```python
from build123d import *

# Parameters (mm, degrees)
SKETCH_1_W          = 145
SKETCH_1_H          = 130
SKETCH_1_R          = 2.25
SKETCH_1_W_2        = 31
SKETCH_1_H_2        = 16
EXTRUDE_1_DEPTH     = 2
SKETCH_2_R          = 0.5
SKETCH_2_R_2        = 0.8
CUT_EXTRUDE_1_DEPTH = 2
SKETCH_3_R          = 1
SKETCH_3_R_2        = 4
SKETCH_3_R_3        = 0.9
CUT_EXTRUDE_2_DEPTH = 2
SKETCH_4_R          = 7.5
SKETCH_4_R_2        = 2.5
SKETCH_4_W          = 29
SKETCH_4_H          = 5
EXTRUDE_2_DEPTH     = 8
SKETCH_5_R          = 0.55
SKETCH_5_R_2        = 0.25
CUT_EXTRUDE_3_DEPTH = 10
SKETCH_6_W          = 27
SKETCH_6_H          = 15
SKETCH_6_W_2        = 7.5
SKETCH_6_H_2        = 18
EXTRUDE_3_DEPTH     = 15
SKETCH_7_W          = 27
SKETCH_7_H          = 15
EXTRUDE_4_DEPTH     = 12
SKETCH_9_R          = 0.3
EXTRUDE_5_DEPTH     = 6.5
EXTRUDE_6_DEPTH     = 0.5
SKETCH_11_R         = 2.45
EXTRUDE_7_DEPTH     = 8.5
CHAMFER_1_SIZE      = 0.5
CHAMFER_1_SIZE2     = 0.08816349


with BuildPart() as part:
    # Эскиз1 → Вытянуть1 (new body)
    with BuildSketch(Plane.XY):
        Rectangle(SKETCH_1_W, SKETCH_1_H)
        with Locations((-67.5, 60)):
            Circle(SKETCH_1_R, mode=Mode.SUBTRACT)
        with Locations((-67.5, -60)):
            Circle(SKETCH_1_R, mode=Mode.SUBTRACT)
        with Locations((67.5, 60)):
            Circle(SKETCH_1_R, mode=Mode.SUBTRACT)
        with Locations((67.5, -60)):
            Circle(SKETCH_1_R, mode=Mode.SUBTRACT)
        with Locations((-52, 20)):
            Rectangle(SKETCH_1_W_2, SKETCH_1_H_2, mode=Mode.SUBTRACT)
        with Locations((-52, -20)):
            Rectangle(SKETCH_1_W_2, SKETCH_1_H_2, mode=Mode.SUBTRACT)
        with Locations((8, 20)):
            Rectangle(SKETCH_1_W_2, SKETCH_1_H_2, mode=Mode.SUBTRACT)
        with Locations((8, -20)):
            Rectangle(SKETCH_1_W_2, SKETCH_1_H_2, mode=Mode.SUBTRACT)
    extrude(amount=EXTRUDE_1_DEPTH)

    # Эскиз2 → Вырез-Вытянуть1 (cut)
    with BuildSketch(Plane.XY.offset(2)):
        with Locations((-57.5, 61)):
            Circle(SKETCH_2_R)
        with Locations((-48, 61)):
            Circle(SKETCH_2_R)
        with Locations((-57.5, 38)):
            Circle(SKETCH_2_R)
        with Locations((-48, 36)):
            Circle(SKETCH_2_R)
        with Locations((-38, 61)):
            Circle(SKETCH_2_R)
        with Locations((-38, 36)):
            Circle(SKETCH_2_R)
        with Locations((-28, 61)):
            Circle(SKETCH_2_R)
        with Locations((-28, 36)):
            Circle(SKETCH_2_R)
        with Locations((-18, 61)):
            Circle(SKETCH_2_R)
        with Locations((-18, 36)):
            Circle(SKETCH_2_R)
        with Locations((-8.5, 61)):
            Circle(SKETCH_2_R)
        with Locations((-8.5, 38)):
            Circle(SKETCH_2_R)
        with Locations(Location((-8.5, -38.5, 0), (0, 0, 180))):
            Circle(SKETCH_2_R)
        with Locations(Location((-8.5, -61.5, 0), (0, 0, 180))):
            Circle(SKETCH_2_R)
        with Locations(Location((-18, -61.5, 0), (0, 0, 180))):
            Circle(SKETCH_2_R)
        with Locations(Location((-18, -36.5, 0), (0, 0, 180))):
            Circle(SKETCH_2_R)
        with Locations(Location((-28, -36.5, 0), (0, 0, 180))):
            Circle(SKETCH_2_R)
        with Locations(Location((-28, -61.5, 0), (0, 0, 180))):
            Circle(SKETCH_2_R)
        with Locations(Location((-38, -61.5, 0), (0, 0, 180))):
            Circle(SKETCH_2_R)
        with Locations(Location((-38, -36.5, 0), (0, 0, 180))):
            Circle(SKETCH_2_R)
        with Locations(Location((-48, -36.5, 0), (0, 0, 180))):
            Circle(SKETCH_2_R)
        with Locations(Location((-48, -61.5, 0), (0, 0, 180))):
            Circle(SKETCH_2_R)
        with Locations(Location((-57.5, -61.5, 0), (0, 0, 180))):
            Circle(SKETCH_2_R)
        with Locations(Location((-57.5, -38.5, 0), (0, 0, 180))):
            Circle(SKETCH_2_R)
        with Locations((-29.5, 20)):
            Circle(SKETCH_2_R_2)
        with Locations((-29.5, -20)):
            Circle(SKETCH_2_R_2)
        with Locations((-29.5, 14.55)):
            Circle(SKETCH_2_R_2)
        with Locations((-29.5, 25.45)):
            Circle(SKETCH_2_R_2)
        with Locations((-29.5, -14.55)):
            Circle(SKETCH_2_R_2)
        with Locations((-29.5, -25.45)):
            Circle(SKETCH_2_R_2)
        with Locations((-14.5, 20)):
            Circle(SKETCH_2_R_2)
        with Locations((-14.5, -20)):
            Circle(SKETCH_2_R_2)
        with Locations((-14.5, 14.55)):
            Circle(SKETCH_2_R_2)
        with Locations((-14.5, 25.45)):
            Circle(SKETCH_2_R_2)
        with Locations((-14.5, -14.866018045)):
            Circle(SKETCH_2_R_2)
        with Locations((-14.5, -25.45)):
            Circle(SKETCH_2_R_2)
    extrude(amount=-CUT_EXTRUDE_1_DEPTH, mode=Mode.SUBTRACT)

    # Эскиз3 → Вырез-Вытянуть2 (cut)
    with BuildSketch(Plane.XY.offset(2)):
        with Locations((13.5, 41.5)):
            Circle(SKETCH_3_R)
        with Locations((13.5, 51.5)):
            Circle(SKETCH_3_R)
        with Locations((49.5, 41.5)):
            Circle(SKETCH_3_R)
        with Locations((49.5, 51.5)):
            Circle(SKETCH_3_R)
        with Locations((13.5, -52)):
            Circle(SKETCH_3_R)
        with Locations((13.5, -42)):
            Circle(SKETCH_3_R)
        with Locations((49.5, -52)):
            Circle(SKETCH_3_R)
        with Locations((49.5, -42)):
            Circle(SKETCH_3_R)
        with Locations((59, 23)):
            Circle(SKETCH_3_R_2)
        with Locations((-68.5, 0)):
            Circle(SKETCH_3_R_3)
        with Locations((-63.42, 0)):
            Circle(SKETCH_3_R_3)
        with Locations((56.5, 14.5)):
            Circle(SKETCH_3_R_3)
        with Locations((61.58, 14.5)):
            Circle(SKETCH_3_R_3)
    extrude(amount=-CUT_EXTRUDE_2_DEPTH, mode=Mode.SUBTRACT)

    # Эскиз4 → Вытянуть2 (add)
    # profile 1 of 3: a face of its own
    with BuildSketch(Plane.XY.offset(2)):
        with Locations(Location((11, -2.5, 0), (0, 0, 180))):
            Circle(SKETCH_4_R)
        with Locations((11, -2.5)):
            Circle(SKETCH_4_R_2, mode=Mode.SUBTRACT)
    # profile 2 of 3: a face of its own
    with BuildSketch(Plane.XY.offset(2)):
        with Locations((-15, 7.5)):
            Rectangle(SKETCH_4_W, SKETCH_4_H)
    # profile 3 of 3: a face of its own
    with BuildSketch(Plane.XY.offset(2)):
        with Locations((-15, -7.5)):
            Rectangle(SKETCH_4_W, SKETCH_4_H)
    extrude(amount=EXTRUDE_2_DEPTH)

    # Эскиз5 → Вырез-Вытянуть3 (cut)
    with BuildSketch(Plane.XY.offset(2)):
        with Locations((33, 5)):
            Circle(SKETCH_5_R)
        with Locations((30.5, -33.5)):
            Circle(SKETCH_5_R_2)
    extrude(amount=-CUT_EXTRUDE_3_DEPTH, mode=Mode.SUBTRACT)

    # Эскиз6 → Вытянуть3 (add)
    with BuildSketch(Plane.XY.offset(2)):
        with Locations((-44, 0)):
            Rectangle(SKETCH_6_W, SKETCH_6_H)
        with Locations((54.25, -19.5)):
            Rectangle(SKETCH_6_W_2, SKETCH_6_H_2)
    extrude(amount=EXTRUDE_3_DEPTH)

    # Эскиз7 → Вытянуть4 (add)
    with BuildSketch(Plane.XY.offset(17)):
        with Locations((-44, 0)):
            Rectangle(SKETCH_7_W, SKETCH_7_H)
    extrude(amount=EXTRUDE_4_DEPTH)

    # Эскиз9 → Вытянуть5 (add)
    with BuildSketch(Plane.XY.offset(2)):
        with Locations((29.23, -32.6)):
            Circle(SKETCH_9_R)
        with Locations((31.77, -32.6)):
            Circle(SKETCH_9_R)
        with Locations((30.5, -34.7)):
            Circle(SKETCH_9_R)
    extrude(amount=-EXTRUDE_5_DEPTH)

    # Эскиз10 → Вытянуть6 (add)
    with BuildSketch(Plane(origin=(0, 0, -4.5), x_dir=(-1, 0, 0), z_dir=(0, 0, -1))):
        with BuildLine():
            Line((-31.84079253, -31.099005333), (-29.15920747, -31.099005333))
            ThreePointArc((-29.15920747, -31.099005333), (-30.5, -36.25), (-31.84079253, -31.099005333))
        make_face()
    extrude(amount=EXTRUDE_6_DEPTH)

    # Эскиз11 → Вытянуть7 (add)
    with BuildSketch(Plane(origin=(0, 0, -5), x_dir=(-1, 0, 0), z_dir=(0, 0, -1))):
        with Locations(Location((-30.5, -33.5, 0), (0, 0, 101.478967652))):
            Circle(SKETCH_11_R)
    extrude(amount=EXTRUDE_7_DEPTH)

    # Фаска1
    chamfer_1_edges = [part.edges().sort_by_distance(p)[0] for p in [
        (30.012429894, -35.900994667, -13.5),
    ]]
    chamfer_1_side = [part.faces().sort_by_distance(p)[0] for p in [
        (30.012429894, -35.900994667, -9.25),
    ]]
    chamfer(chamfer_1_edges, length=CHAMFER_1_SIZE, length2=CHAMFER_1_SIZE2, reference=chamfer_1_side[0])


solid = part.part
```
Model file for the job. Use its own axes, mm. A direction names the side the tool comes from. Coordinates: 2 decimals unless noted, no trailing zeros. Order: outer loops, then holes, each group sorted by start corner. A loop starts at its lowest first (then second) coordinate and runs counter-clockwise, first axis right, second up. Notation, with made-up numbers: (68, 16.5) -> (90, 16.5) arc R22 cw to (90, 26.5) -> close; hole circle Ø11 at (31.25, -9.5). An arc over 180 degrees is marked (long way). Answer as a JSON object with one key per item and string values. Group by question number.
1) Drill centre lines: L1, parallel to X at y = 38, z = 1.25; L2, parallel to Y at x = -18, z = 1; L3, parallel to Y at x = 49.5, z = 0.85. Where is each one in solid material? Low to high.
2) Which spindle directions (+Z, -Z, +X, -X, +Y, -Y) get a long thin tool onto all of the face, cutting with end or side? Do faces 4 (the face through (-15, 10, 6)), 5 (the face through (54, -28.5, 9)), 6 (the face through (11, 1, 10)), 7 (the face through (50.5, -20, 9)). Say none if no direction does.
3) Pull direction Y, two halves, no side cores. Call faces 1 (the face through (11, -2, 2)), 2 (the face through (31.69, -31.36, -8.94)), 3 (the face through (-44, 7.5, 15)): +Y half, -Y half, draft (parallel to the pull), parting line (faces both ways), or undercut.
4) Cut at C-C, the plane z = -11. Write the cut outline in (x, y), then the cut area to 3 significant figures.
5) Cut at B-B, the plane y = -23. Write the cut outline in (x, z).
6) Flat gauge pins, fed straight in: pin 1 (10 mm diameter, centred on x = -57.5, z = 10.5, fed in from -Y); pin 2 (7 mm diameter, centred on x = 67.5, y = 60, fed in from -Z); pin 3 (12 mm diameter, centred on x = -20.5, y = -29.5, fed in from +Z). Where does each tip first touch, or does it go through?
7) Cut at A-A, the plane x = -51. Write the cut outline in (y, z), then the cut area to 3 significant figures.
Check values:
{
 "1": {"L1": "x = -72.5 to -58, -57 to -9, -8 to 72.5", "L2": "y = -65 to -62, -61 to -37, -36 to 35.5, 36.5 to 60.5, 61.5 to 65", "L3": "y = -65 to -53, -51 to -43, -41 to 40.5, 42.5 to 50.5, 52.5 to 65"},
 "2": {"face 4": "+Z, +X, -X, +Y", "face 5": "+Z, +X, -X, -Y", "face 6": "+Z, +X, +Y, -Y", "face 7": "+Z, -X, +Y, -Y"},
 "3": {"face 1": "undercut", "face 2": "parting line", "face 3": "+Y half"},
 "4": {"outline": "circle Ø4.9 at (30.5, -33.5)", "area": "18.9 mm²"},
 "5": {"outline": "(-72.5, 0) -> (-67.5, 0) -> (-67.5, 2) -> (-72.5, 2) -> close; (-36.5, 0) -> (-7.5, 0) -> (-7.5, 2) -> (-36.5, 2) -> close; (23.5, 0) -> (72.5, 0) -> (72.5, 2) -> (58, 2) -> (58, 17) -> (50.5, 17) -> (50.5, 2) -> (23.5, 2) -> close"},
 "6": {"pin 1": "stops at y = -7.5", "pin 2": "stops at z = 0", "pin 3": "stops at z = 2"},
 "7": {"outline": "(-65, 0) -> (-28, 0) -> (-28, 2) -> (-65, 2) -> close; (-12, 0) -> (12, 0) -> (12, 2) -> (7.5, 2) -> (7.5, 29) -> (-7.5, 29) -> (-7.5, 2) -> (-12, 2) -> close; (28, 0) -> (65, 0) -> (65, 2) -> (28, 2) -> close", "area": "601 mm²"}
}
